The model under review builds one solid part; all positions refer to its coordinate system, in mm. Face numbers are marked on the shaded views. A direction names the side the tool comes from. Coordinates: 2 decimals unless noted, no trailing zeros. Loops run counter-clockwise (first coordinate to the right, second up) from the corner with the lowest first, then second, coordinate; pieces in that order, holes last. Notation, with made-up numbers: M -37.75,-25 L -14.75,-25 A16 cw -14.75,-3 Z; hole C 2,-32.5 d3. An arc over 180 degrees is marked long. Write item = value, one per line. Start each with the question number.
Q1. We need section B-B on y = 98. Give the boundary of the cut face in (x, z), and give its area (3 significant figures).
Q2. We need section A-A on z = -118.75. Count the separate pieces of the cut face and the enclosed holes in it, and give its area (3 significant figures).
Q3. We need section C-C on x = -31.75. Give the boundary of the cut face in (y, z).
Q4. Mouldability with a two-part tool opening along X and no side actions: class the marked faces 4, 5, 6 and 7 as released by +X, released by -X, zero draft, split by the parting line, or undercut.
Q5. Clearance check with flat-ended pins moving along their axes: pin 1 Ø2 at (x, z) = (-32.5, -122) entering from +Y; pin 2 Ø3 at (x, z) = (-26, -120) entering from +Y; pin 3 Ø2.5 at (y, z) = (106, -120) entering from -X; pin 4 Ø4 at (x, y) = (-34, 85) entering from +Z. State where each tip first meets the part, or that it passes through.
Q6. For the marked faces 1, 2 and 3, list the 3-axis set-ups (+Z, -Z, +X, -X, +Y, -Y) from which the entire face can be reached by the end or side of a thin tool; tool diameter is ignored.
Q7. Wall thickness on probe 1 along X at (y, z) = (104.5, -119.25); probe 2 along Y at (x, z) = (-32.25, -119.5); probe 3 along Z at (x, y) = (-28.25, 82): over which ranges is each line inside the solid? List them lowest first.
Q8. We need section D-D on z = -121.75. Give the boundary of the cut face in (x, y).
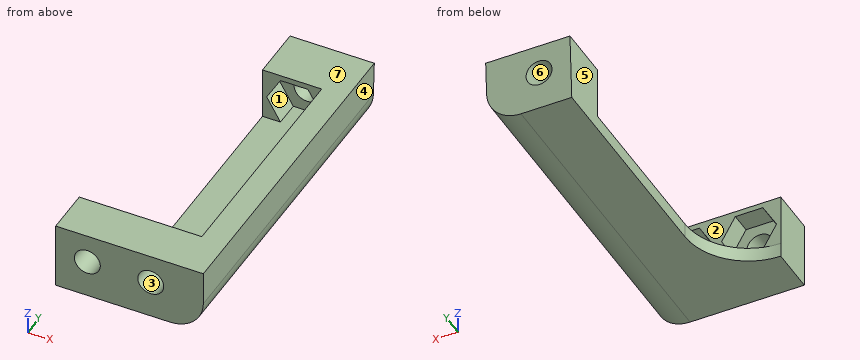
from build123d import *

# Parameters (mm, degrees)
SKETCH4_R                 = 1.55
BOSS_EXTRUDE4_DEPTH       = 3
BOSS_EXTRUDE5_START       = 3
BOSS_EXTRUDE5_DEPTH       = 2.5
BOSS_EXTRUDE6_START       = 5.5
BOSS_EXTRUDE6_DEPTH       = 31.423000022
BOSS_EXTRUDE6_START_2     = 116.532620121
BOSS_EXTRUDE6_2_OUTLINE_W = 13
BOSS_EXTRUDE6_2_OUTLINE_H = 11
BOSS_EXTRUDE6_2_DEPTH     = 1.467379879
BOSS_EXTRUDE7_START       = 36.497247904
BOSS_EXTRUDE7_OUTLINE_R   = 1.55
BOSS_EXTRUDE7_DEPTH       = 3.429880261
BOSS_EXTRUDE7_START_2     = 119.532620121
BOSS_EXTRUDE7_2_OUTLINE_W = 13
BOSS_EXTRUDE7_2_OUTLINE_H = 12
BOSS_EXTRUDE7_2_DEPTH     = 1.467379879
BOSS_EXTRUDE8_START       = 33.497248
BOSS_EXTRUDE8_DEPTH       = 3
SKETCH4_12_W              = 7.581793069
SKETCH4_12_H              = 8.112892266
SKETCH4_12_R              = 1.55
BOSS_EXTRUDE10_DEPTH      = 3
BOSS_EXTRUDE11_START      = 3
SKETCH4_13_W              = 7.581793069
SKETCH4_13_H              = 8.112892266
BOSS_EXTRUDE11_DEPTH      = 2.5
BOSS_EXTRUDE12_DEPTH      = 1.75


with BuildPart() as part:
    # Sketch4 → Boss-Extrude4 (new body)
    with BuildSketch(Plane(origin=(0, 73.681369419, 0), x_dir=(1, 0, 0), z_dir=(0, 1, 0))):
        with BuildLine():
            Line((-30.198456841, 124.133918355), (-24.116663772, 124.133918355))
            ThreePointArc((-24.116663772, 124.133918355), (-21.288236648, 122.96234548), (-20.116663772, 120.133918355))
            Line((-20.116663772, 120.133918355), (-20.116663772, 116.021026089))
            Line((-20.116663772, 116.021026089), (-30.198456841, 116.021026089))
            Line((-30.198456841, 116.021026089), (-30.198456841, 124.133918355))
        make_face()
        with Locations(Location((-26.407560307, 119.533918355, 0), (0, 0, 180))):
            Circle(SKETCH4_R, mode=Mode.SUBTRACT)
    extrude(amount=BOSS_EXTRUDE4_DEPTH)

    # Sketch4<5> → Boss-Extrude5 (add)
    with BuildSketch(Plane(origin=(0, 73.681369419, 0), x_dir=(1, 0, 0), z_dir=(0, 1, 0)).offset(BOSS_EXTRUDE5_START)):
        with BuildLine():
            Line((-24.116663772, 124.133918355), (-30.198456841, 124.133918355))
            Line((-30.198456841, 124.133918355), (-30.198456841, 122.383918355))
            Line((-30.198456841, 122.383918355), (-28.053008574, 122.383918355))
            Line((-28.053008574, 122.383918355), (-24.762112039, 122.383918355))
            Line((-24.762112039, 122.383918355), (-23.116663772, 119.533918355))
            Line((-23.116663772, 119.533918355), (-23.116663772, 116.021026089))
            Line((-23.116663772, 116.021026089), (-20.116663772, 116.021026089))
            Line((-20.116663772, 116.021026089), (-20.116663772, 120.133918355))
            ThreePointArc((-20.116663772, 120.133918355), (-21.288236648, 122.96234548), (-24.116663772, 124.133918355))
        make_face()
        Polygon((-28.053008574, 122.383918355), (-30.198456841, 122.383918355), (-30.198456841, 116.021026089), (-23.116663772, 116.021026089), (-23.116663772, 119.533918355), (-24.762112039, 116.683918355), (-28.053008574, 116.683918355), (-29.698456841, 119.533918355), align=None)
    extrude(amount=BOSS_EXTRUDE5_DEPTH)

    # Boss-Extrude6: read off the stored shape, not the designer's step
    # Boss-Extrude6 outline → Boss-Extrude6 (add)
    with BuildSketch(Plane(origin=(0, 73.681369419, 0), x_dir=(1, 0, 0), z_dir=(0, 1, 0)).offset(BOSS_EXTRUDE6_START)):
        with BuildLine():
            Line((-24.116663772, 124.133918355), (-30.198456841, 124.133918355))
            Line((-30.198456841, 124.133918355), (-30.198456841, 122.383918355))
            Line((-30.198456841, 122.383918355), (-24.762112039, 122.383918355))
            Line((-24.762112039, 122.383918355), (-23.116663772, 119.533918355))
            Line((-23.116663772, 119.533918355), (-23.116663772, 116.021026089))
            Line((-23.116663772, 116.021026089), (-20.116663772, 116.021026089))
            Line((-20.116663772, 116.021026089), (-20.116663772, 120.133918355))
            ThreePointArc((-20.116663772, 120.133918355), (-21.288236648, 122.96234548), (-24.116663772, 124.133918355))
        make_face()
    extrude(amount=BOSS_EXTRUDE6_DEPTH)

    # Boss-Extrude6 2 outline → Boss-Extrude6 2 (cut)
    with BuildSketch(Plane(origin=(0, 0, 0), x_dir=(1, 0, 0), z_dir=(0, 0.9986258431157963, -0.05240634943654381)).offset(BOSS_EXTRUDE6_START_2)):
        with Locations((-25.5, 114.5)):
            Rectangle(BOSS_EXTRUDE6_2_OUTLINE_W, BOSS_EXTRUDE6_2_OUTLINE_H)
    extrude(amount=BOSS_EXTRUDE6_2_DEPTH, mode=Mode.SUBTRACT)

    # Boss-Extrude7: read off the stored shape, not the designer's step
    # Boss-Extrude7 outline → Boss-Extrude7 (add)
    with BuildSketch(Plane(origin=(0, 73.681369419, 0), x_dir=(1, 0, 0), z_dir=(0, 1, 0)).offset(BOSS_EXTRUDE7_START)):
        with BuildLine():
            Line((-30.198456841, 116.021026089), (-20.116663772, 116.021026089))
            Line((-20.116663772, 116.021026089), (-20.116663772, 120.133918355))
            ThreePointArc((-20.116663772, 120.133918355), (-21.288236648, 122.96234548), (-24.116663772, 124.133918355))
            Line((-24.116663772, 124.133918355), (-30.198456841, 124.133918355))
            Line((-30.198456841, 124.133918355), (-30.198456841, 116.021026089))
        make_face()
        with Locations((-26.407560307, 119.533918355)):
            Circle(BOSS_EXTRUDE7_OUTLINE_R, mode=Mode.SUBTRACT)
    extrude(amount=BOSS_EXTRUDE7_DEPTH)

    # Boss-Extrude7 2 outline → Boss-Extrude7 2 (cut)
    with BuildSketch(Plane(origin=(0, 0, 0), x_dir=(1, 0, 0), z_dir=(0, 0.9986258431157963, -0.05240634943654381)).offset(BOSS_EXTRUDE7_START_2)):
        with Locations((-25.5, 114)):
            Rectangle(BOSS_EXTRUDE7_2_OUTLINE_W, BOSS_EXTRUDE7_2_OUTLINE_H)
    extrude(amount=BOSS_EXTRUDE7_2_DEPTH, mode=Mode.SUBTRACT)

    # Sketch4<10> → Boss-Extrude8 (add)
    with BuildSketch(Plane(origin=(0, 73.681369419, 0), x_dir=(1, 0, 0), z_dir=(0, 1, 0)).offset(BOSS_EXTRUDE8_START)):
        with BuildLine():
            Line((-24.116663772, 124.133918355), (-30.198456841, 124.133918355))
            Line((-30.198456841, 124.133918355), (-30.198456841, 122.383918355))
            Line((-30.198456841, 122.383918355), (-28.053008574, 122.383918355))
            Line((-28.053008574, 122.383918355), (-24.762112039, 122.383918355))
            Line((-24.762112039, 122.383918355), (-23.116663772, 119.533918355))
            Line((-23.116663772, 119.533918355), (-23.116663772, 116.021026089))
            Line((-23.116663772, 116.021026089), (-20.116663772, 116.021026089))
            Line((-20.116663772, 116.021026089), (-20.116663772, 120.133918355))
            ThreePointArc((-20.116663772, 120.133918355), (-21.288236648, 122.96234548), (-24.116663772, 124.133918355))
        make_face()
        Polygon((-28.053008574, 122.383918355), (-30.198456841, 122.383918355), (-30.198456841, 116.021026089), (-23.116663772, 116.021026089), (-23.116663772, 119.533918355), (-24.762112039, 116.683918355), (-28.053008574, 116.683918355), (-29.698456841, 119.533918355), align=None)
    extrude(amount=BOSS_EXTRUDE8_DEPTH)

    # Sketch4<12> → Boss-Extrude10 (add)
    # profile 1 of 2: a face of its own
    with BuildSketch(Plane(origin=(0, 73.681369419, 0), x_dir=(1, 0, 0), z_dir=(0, 1, 0))):
        with Locations((-33.989353376, 120.077472222)):
            Rectangle(SKETCH4_12_W, SKETCH4_12_H)
        Polygon((-32.343905108, 116.683918355), (-30.698456841, 119.533918355), (-32.343905108, 122.383918355), (-35.634801643, 122.383918355), (-37.28024991, 119.533918355), (-35.634801643, 116.683918355), align=None, mode=Mode.SUBTRACT)
    # profile 2 of 2: a face of its own
    with BuildSketch(Plane(origin=(0, 73.681369419, 0), x_dir=(1, 0, 0), z_dir=(0, 1, 0))):
        Polygon((-35.634801643, 116.683918355), (-32.343905108, 116.683918355), (-30.698456841, 119.533918355), (-32.343905108, 122.383918355), (-35.634801643, 122.383918355), (-37.28024991, 119.533918355), align=None)
        with Locations(Location((-33.989353375, 119.533918355, 0), (0, 0, 180))):
            Circle(SKETCH4_12_R, mode=Mode.SUBTRACT)
    extrude(amount=BOSS_EXTRUDE10_DEPTH)

    # Sketch4<13> → Boss-Extrude11 (add)
    with BuildSketch(Plane(origin=(0, 73.681369419, 0), x_dir=(1, 0, 0), z_dir=(0, 1, 0)).offset(BOSS_EXTRUDE11_START)):
        with Locations((-33.989353376, 120.077472222)):
            Rectangle(SKETCH4_13_W, SKETCH4_13_H)
        Polygon((-32.343905108, 116.683918355), (-30.698456841, 119.533918355), (-32.343905108, 122.383918355), (-35.634801643, 122.383918355), (-37.28024991, 119.533918355), (-35.634801643, 116.683918355), align=None, mode=Mode.SUBTRACT)
    extrude(amount=BOSS_EXTRUDE11_DEPTH)

    # Sketch7 → Boss-Extrude12 (add)
    with BuildSketch(Plane(origin=(0, 0, -124.133918355), x_dir=(-1, 0, 0), z_dir=(0, 0, -1))):
        with BuildLine():
            Line((30.198456841, 79.181369419), (37.78024991, 79.181369419))
            ThreePointArc((37.78024991, 79.181369419), (32.419112617, 81.402025196), (30.198456841, 86.763162488))
            Line((30.198456841, 86.763162488), (30.198456841, 79.181369419))
        make_face()
    extrude(amount=-BOSS_EXTRUDE12_DEPTH)


solid = part.part
Returned:
q1.outline = M -30.2,-124.13 L -24.12,-124.13 A4 ccw -20.12,-120.13 L -20.12,-116.02 L -23.12,-116.02 L -23.12,-119.53 L -24.76,-122.38 L -30.2,-122.38 Z
q1.area = 35.6 mm^2
q2.separate_pieces = 4
q2.enclosed_holes = 0
q2.area = 174 mm^2
q3.outline = M 73.68,-124.13 L 82.17,-124.13 L 82.17,-122.38 L 79.18,-122.38 L 79.18,-121.36 L 76.68,-121.36 L 76.68,-117.71 L 79.18,-117.71 L 79.18,-116.02 L 73.68,-116.02 Z
q4.face_4 = released by +X
q4.face_5 = released by -X
q4.face_6 = undercut
q4.face_7 = zero draft
q5.pin_1 = 82.4
q5.pin_2 = 113.46
q5.pin_3 = -30.2
q5.pin_4 = through
q6.face_1 = none
q6.face_2 = +Z, -X
q6.face_3 = +Y, -Y
q7.probe_1 = -23.12 to -20.12
q7.probe_2 = 73.68 to 76.68
q7.probe_3 = -124.13 to -122.38
q8.outline = M -37.78,73.68 L -20.46,73.68 L -20.46,113.31 L -30.2,113.31 L -30.2,107.18 L -28.42,107.18 L -28.42,110.18 L -24.4,110.18 L -24.4,76.68 L -28.42,76.68 L -28.42,79.18 L -31.98,79.18 L -31.98,76.68 L -36,76.68 L -36,79.18 L -37.78,79.18 Z
